Autodesk Inventor part; units mm, degrees
ref_plane "РабПлоскость1" through (15, 0, 0) normal (1, 0, 0) x (0, 1, 0)
ref_plane "XZ Plane" through (0, 0, 0) normal (0, 1, 0) x (-1, 0, 0)
ref_plane "XY Plane" through (0, 0, 0) normal (0, 0, 1) x (1, 0, 0)
sketch "Эскиз1" plane through (0, 0, 0) normal (1, 0, 0) x (0, 1, 0)
  line L0 (0, 0) -> (0, 9)
  line L1 (0, 9) -> (17.25, 9)
  line L2 (17.25, 9) -> (18.7071, 7.5429)
  line L3 (19.4142, 7.25) -> (23.4, 7.25)
  line L4 (25, 8.85) -> (25, 15)
  line L5 (25, 15) -> (65, 15)
  line L6 (65, 15) -> (65, 10)
  line L7 (65, 10) -> (95, 10)
  line L8 (95, 0) -> (0, 0)
  line L9 (95, 10) -> (95, 0)
  arc A0 (18.7071, 7.5429) -> (19.4142, 7.25) centre (19.4142, 8.25) ccw
  arc A1 (23.4, 7.25) -> (25, 8.85) centre (23.4, 8.85) ccw
  point P0 (19, 7.25)
  point P1 (25, 7.25)
  dimension "d0" = 95
  dimension "d1" = 18
  dimension "d2" = 14.5
  dimension "d3" = 45
  dimension "d4" = 40
  dimension "d5" = 25
  dimension "d6" = 6
  dimension "d7" = 20
  dimension "d8" = 30
  dimension "d9" = 1
  dimension "d10" = 1.6
revolve "Вращение1" add sketch "Эскиз1" angle 360 about axis through (0, 95, 0) along (0, -1, 0)
thread "Резьба1"
chamfer "Фаска1" distance 2.5 angle 45 1 edges at (0, 0, -9)
chamfer "Фаска2" distance 1 angle 45 2 edges at (0, 25, -15) (0, 65, -15)
ref_plane "РабПлоскость1" through (15, 0, 0) normal (1, 0, 0) x (0, 1, 0)
sketch "Эскиз2" plane through (15, 0, 0) normal (1, 0, 0) x (0, 1, 0)
  line L0 (25, -14) -> (25, 14)
  point P0 (0, 0)
  point P1 (45, 0)
  dimension "d21" = 20
hole "Отверстие1" at (15, 45, 0) direction (-1, 0, 0) diameter 10 depth 15 tip angle 120
sketch "Эскиз3" plane through (0, 0, 0) normal (1, 0, 0) x (0, 1, 0)
  line L0 (95, 10) -> (75, 10)
  line L1 (75, 10) -> (75, 6.5)
  line L2 (75, 6.5) -> (95, 6.5)
  line L3 (95, 6.5) -> (95, 10)
  line L4 (-19.7495, 0) -> (118.4967, 0)
  line L5 (95, -10) -> (95, 10)
  line L6 (65, 10) -> (95, 10)
  line L7 (-19, 0) -> (114, 0)
  line L8 (95, -10) -> (75, -10)
  line L9 (75, -10) -> (75, -6.5)
  line L10 (75, -6.5) -> (95, -6.5)
  line L11 (95, -6.5) -> (95, -10)
  point P0 (0, 0)
  dimension "d29" = 6.5
  dimension "d30" = 20
extrude "Выдавливание1" cut sketch "Эскиз3" along normal through all both and the other way through all
sketch "Эскиз4" plane through (-7.5993, 95, 6.5) normal (0, 0, 1) x (1, 0, 0)
  line L0 (0, 0) -> (15.1987, 0)
  line L1 (-2.4007, -30) -> (-2.4007, 0)
  point P0 (7.5993, -95)
  point P1 (7.5993, -8)
  dimension "d33" = 10
  dimension "d34" = 8
hole "Отверстие2" at (0, 87, 6.5) direction (0, 0, -1) diameter 4 end through all
properties part number "Вал_19"
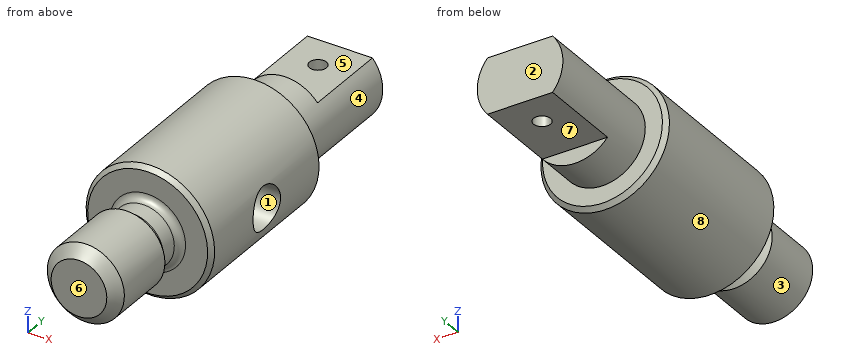
Model file for the job. Use its own axes, mm. Face numbers are marked on the shaded views. A direction names the side the tool comes from. Give positions to 0.01 mm unless a question says otherwise; leave off trailing zeros. Order: outer loops, then holes, each group sorted by start corner. A loop starts at its lowest first (then second) coordinate and runs counter-clockwise, first axis right, second up. Notation, with made-up numbers: (-15, 62.5) - (26, 62.5) arc R20 ccw to (26, 86.5) - close; hole circle Ø8 at (-22.5, 57.5). An arc over 180 degrees is marked (long way). Write item = value, one per line. Start each with the question number.
1. Cut at C-C, the plane y = 71.5. List the corners of the cut face in (x, z).
2. Cut at B-B, the plane y = 32.5. List the corners of the cut face in (x, z), and give its area (3 significant figures).
3. Two-plate mould, pull along Z, no slides. Class the marked faces 1, 2 and 3: pulls with the +Z half, pulls with the -Z half, needs draft (parallel to the pull), parting line crosses it, or undercut.
4. Drop flat-ended pins along their axis: P1, Ø5, axis at x = 0, y = 87, coming from the -Z side; P2, Ø1, axis at x = -1.5, y = 54.5, coming from the -Z side; P3, Ø1, axis at x = 1.5, z = 8, coming from the +Y side. Give the stop position or say it passes through.
5. Probe line 1 along Y through (x, z) = (11, 0); line 2 along Y through (x, z) = (0, -0.5); line 3 along Y through (x, z) = (0, -3). List the from-to ranges inside material, lowest first.
6. Which spindle directions (+Z, -Z, +X, -X, +Y, -Y) get a long thin tool onto all of the face, cutting with end or side? Do the marked faces 4, 5, 6, 7 and 8. Say none if no direction does.
7. Cut at A-A, the plane y = 87. List the corners of the cut face in (x, z), and give its area (3 significant figures).
Taken from the geometry:
q1.outline = circle Ø20 at (0, 0)
q2.outline = circle Ø30 at (0, 0)
q2.area = 707 mm²
q3.face_1 = undercut
q3.face_2 = needs draft
q3.face_3 = parting line crosses it
q4.P1 = -6.5
q4.P2 = -14.97
q4.P3 = 75
q5.line_1 = 25 to 40, 50 to 65
q5.line_2 = 0 to 40.03, 49.97 to 85, 89 to 95
q5.line_3 = 0 to 41, 49 to 85, 89 to 95
q6.face_4 = +Y
q6.face_5 = +Z, +X, -X, +Y
q6.face_6 = +Z, -Z, +X, -X, -Y
q6.face_7 = -Z, +X, -X, +Y
q6.face_8 = +Y, -Y
q7.outline = (-7.6, -6.5) - (-2, -6.5) - (-2, 6.5) - (-7.6, 6.5) arc R10 ccw to start; (2, -6.5) - (7.6, -6.5) arc R10 ccw to (7.6, 6.5) - (2, 6.5) - close
q7.area = 188 mm²
